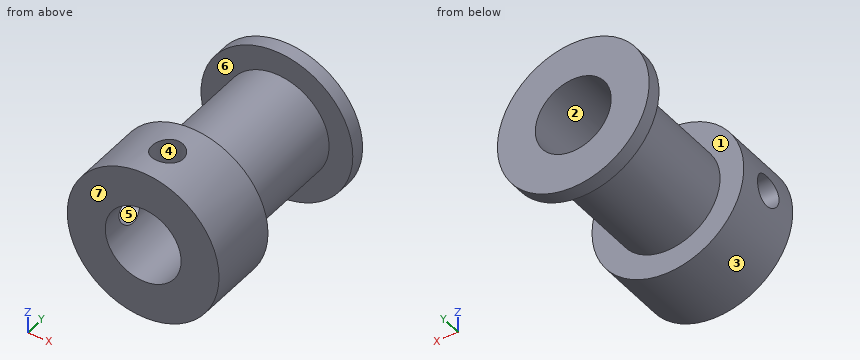
from build123d import *

# Parameters (mm, degrees)
CROQUIS1_R              = 8
SALIENTE_EXTRUIR1_DEPTH = 7.5
CROQUIS2_R              = 5.5
SALIENTE_EXTRUIR2_DEPTH = 13
CROQUIS3_R              = 8
SALIENTE_EXTRUIR3_DEPTH = 1.5
CROQUIS4_R              = 4
CORTAR_EXTRUIR1_DEPTH   = 23
CROQUIS6_W              = 1.65
CROQUIS6_H              = 8.001
MATRIZC1_COUNT          = 2
MATRIZC1_ANGLE          = 90


with BuildPart() as part:
    # Croquis1 → Saliente-Extruir1 (new body)
    with BuildSketch(Plane(origin=(0, 0, 0), x_dir=(1, 0, 0), z_dir=(0, 1, 0))):
        Circle(CROQUIS1_R)
    extrude(amount=SALIENTE_EXTRUIR1_DEPTH)

    # Croquis2 → Saliente-Extruir2 (add)
    with BuildSketch(Plane(origin=(0, 7.5, 0), x_dir=(1, 0, 0), z_dir=(0, 1, 0))):
        Circle(CROQUIS2_R)
    extrude(amount=SALIENTE_EXTRUIR2_DEPTH)

    # Croquis3 → Saliente-Extruir3 (add)
    with BuildSketch(Plane(origin=(0, 20.5, 0), x_dir=(1, 0, 0), z_dir=(0, 1, 0))):
        Circle(CROQUIS3_R)
    extrude(amount=SALIENTE_EXTRUIR3_DEPTH)

    # Croquis4 → Cortar-Extruir1 (cut, through all)
    with BuildSketch(Plane(origin=(0, 22, 0), x_dir=(1, 0, 0), z_dir=(0, 1, 0))):
        Circle(CROQUIS4_R)
    extrude(amount=-CORTAR_EXTRUIR1_DEPTH, mode=Mode.SUBTRACT)

    # Croquis6 → Taladro roscado M41 (falta definir posicio) (revolve, cut)
    with BuildSketch(Plane(origin=(0, 3.75, 0), x_dir=(0, 1, 0), z_dir=(1, 0, 0))):
        with Locations((0.825, 4.0005)):
            Rectangle(CROQUIS6_W, CROQUIS6_H)
    taladro_roscado_m41_falta_definir_posic = revolve(axis=Axis((0, 3.75, -6.35), (0, 0, 1)), mode=Mode.SUBTRACT)

    # MatrizC1: Taladro roscado M41 (falta definir posicio) ×2 about axis
    matrizc1_axis = Axis((0, 7.5, 0), (0, -1, 0))
    for i in range(1, MATRIZC1_COUNT):
        add(taladro_roscado_m41_falta_definir_posic.rotate(matrizc1_axis, i * MATRIZC1_ANGLE / (MATRIZC1_COUNT - 1)), mode=Mode.SUBTRACT)


solid = part.part
The listing builds one solid part. Answer for the finished solid, in the listing's coordinates (mm). Face numbers are marked on the shaded views. A direction names the side the tool comes from. Give positions to 0.01 mm unless a question says otherwise; leave off trailing zeros. Write each loop counter-clockwise with the first axis right and the second up, starting at its lowest first coordinate (ties: lowest second). Pieces come first, ordered by that corner, then holes. Notation, with made-up numbers: (3.25, -11) - (12.25, -11) arc R18 ccw to (12.25, 1) - close; hole circle Ø8 at (75.25, 17.5). An arc over 180 degrees is marked (long way). One line per question, with ' | ' between items. Start each with the question number.
1. Given P1, Ø1.5, axis at x = -5.5, y = 13.5, coming from the -Z side; P2, Ø4, axis at x = -5, y = 12.5, coming from the +Z side; P3, Ø2, axis at x = 0, y = 3.75, coming from the +Z side, each flat-ended and moving along its own axis, determine where each tip first touches the part or whether it passes through.
2. Determine the mould class of the marked faces 1, 2 and 3 for opening direction Z: +Z half, -Z half, draft (parallel to the pull), parting line (faces both ways), or undercut.
3. Section D-D, the plane y = 3.75 is taken. Determine the outline of the cut face in (x, z), then the cut area to 3 significant figures.
4. For the marked faces 4, 5, 6 and 7, determine the directions among +Z, -Z, +X, -X, +Y, -Y from which every point of the face is accessible in a straight line to the end or side of a thin tool.
5. Section C-C, the plane x = 0 is taken. Determine the outline of the cut face in (y, z).
6. Section B-B, the plane z = 0 is taken. Determine the outline of the cut face in (x, y), then the cut area to 3 significant figures.
7. Straight lines are drawn through the part: line 1 (Y direction, x = 0, z = 6.6); line 2 (X direction, y = 12.5, z = 0); line 3 (Y direction, x = -3.5, z = 5.5). For each, find the intervals that lie inside material, in ascending order.
8. Section A-A, the plane x = -6 is taken. Determine the outline of the cut face in (y, z), then the cut area to 3 significant figures.
Result:
1) P1: stops at z = -2.77 | P2: stops at z = 4.61 | P3: stops at z = -3.87
2) face 1: draft | face 2: undercut | face 3: parting line
3) outline: (-7.83, -1.65) arc R8 ccw (long way) to (1.65, 7.83) - (1.65, 3.64) arc R4 cw (long way) to (-3.64, -1.65) - close; (-7.83, 1.65) - (-3.64, 1.65) arc R4 cw to (-1.65, 3.64) - (-1.65, 7.83) arc R8 ccw to start | area: 124 mm2
4) face 4: +Z | face 5: -X | face 6: none | face 7: +Z, -Z, +X, -X, -Y
5) outline: (0, -8) - (7.5, -8) - (7.5, -5.5) - (20.5, -5.5) - (20.5, -8) - (22, -8) - (22, -4) - (0, -4) - close; (0, 4) - (2.1, 4) - (2.1, 8) - (0, 8) - close; (5.4, 4) - (22, 4) - (22, 8) - (20.5, 8) - (20.5, 5.5) - (7.5, 5.5) - (7.5, 8) - (5.4, 8) - close
6) outline: (-8, 0) - (-4, 0) - (-4, 2.1) - (-8, 2.1) - close; (-8, 5.4) - (-4, 5.4) - (-4, 22) - (-8, 22) - (-8, 20.5) - (-5.5, 20.5) - (-5.5, 7.5) - (-8, 7.5) - close; (4, 0) - (8, 0) - (8, 7.5) - (5.5, 7.5) - (5.5, 20.5) - (8, 20.5) - (8, 22) - (4, 22) - close | area: 97.8 mm2
7) line 1: y = 0 to 2.1, 5.4 to 7.5, 20.5 to 22 | line 2: x = -5.5 to -4, 4 to 5.5 | line 3: y = 0 to 7.5, 20.5 to 22
8) outline: (0, -5.29) - (7.5, -5.29) - (7.5, 5.29) - (0, 5.29) - close; (20.5, -5.29) - (22, -5.29) - (22, 5.29) - (20.5, 5.29) - close; hole circle Ø3.3 at (3.75, 0) | area: 86.7 mm2
